For this review, take the finished solid that the model builds, in its own axes (mm). Face numbers are marked on the shaded views. A direction names the side the tool comes from. Give positions to 0.01 mm unless a question says otherwise; leave off trailing zeros. Loops run counter-clockwise (first coordinate to the right, second up) from the corner with the lowest first, then second, coordinate; pieces in that order, holes last. Notation, with made-up numbers: (-33, 2.5) - (23, 2.5) arc R38 cw to (23, 41.5) - close; hole circle Ø7 at (-35.5, 8.25). An arc over 180 degrees is marked (long way). Answer in a Markdown table with one row per item.
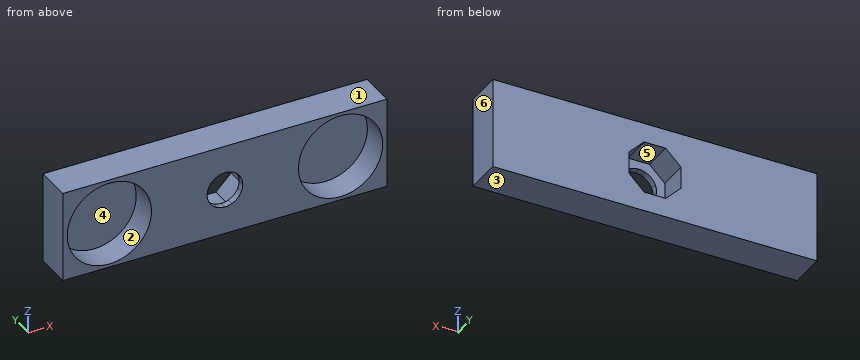
```python
from build123d import *

# Parameters (mm, degrees)
F1_DEPTH = 13.9
F2_DEPTH = 25
F3_R     = 19.5
F4_DEPTH = 17
F6_DEPTH = 20.74372


with BuildPart() as f1:
    # F0 (on Front) → F1 (new body)
    with BuildSketch(Plane.XZ):
        with BuildLine():
            Line((5.0119841047, 12.1), (3.157138317, 7.6220061432))
            ThreePointArc((3.157138317, 7.6220061432), (5.8336309448, 5.8336309448), (7.6220061432, 3.157138317))
            Line((7.6220061432, 3.157138317), (12.1, 5.0119841047))
            Line((12.1, 5.0119841047), (5.0119841047, 12.1))
        make_face()
        with BuildLine():
            Line((0, 12.1), (0, 8.25))
            ThreePointArc((0, 8.25), (1.6094951566, 8.0914785633), (3.157138317, 7.6220061432))
            Line((3.157138317, 7.6220061432), (5.0119841047, 12.1))
            Line((5.0119841047, 12.1), (0, 12.1))
        make_face()
        with BuildLine():
            ThreePointArc((-3.157138317, 7.6220061432), (-1.6094951566, 8.0914785633), (0, 8.25))
            Line((0, 8.25), (0, 12.1))
            Line((0, 12.1), (-5.0119841047, 12.1))
            Line((-5.0119841047, 12.1), (-3.157138317, 7.6220061432))
        make_face()
        with BuildLine():
            ThreePointArc((-7.6220061432, 3.157138317), (-5.8336309448, 5.8336309448), (-3.157138317, 7.6220061432))
            Line((-3.157138317, 7.6220061432), (-5.0119841047, 12.1))
            Line((-5.0119841047, 12.1), (-12.1, 5.0119841047))
            Line((-12.1, 5.0119841047), (-7.6220061432, 3.157138317))
        make_face()
        with BuildLine():
            ThreePointArc((-3.157138317, -7.6220061432), (-5.8336309448, -5.8336309448), (-7.6220061432, -3.157138317))
            Line((-7.6220061432, -3.157138317), (-12.1, -5.0119841047))
            Line((-12.1, -5.0119841047), (-5.0119841047, -12.1))
            Line((-5.0119841047, -12.1), (-3.157138317, -7.6220061432))
        make_face()
        with BuildLine():
            ThreePointArc((-7.6220061432, -3.157138317), (-8.0914785633, -1.6094951566), (-8.25, 0))
            Line((-8.25, 0), (-12.1, 0))
            Line((-12.1, 0), (-12.1, -5.0119841047))
            Line((-12.1, -5.0119841047), (-7.6220061432, -3.157138317))
        make_face()
        with BuildLine():
            Line((-12.1, 0), (-8.25, 0))
            ThreePointArc((-8.25, 0), (-8.0914785633, 1.6094951566), (-7.6220061432, 3.157138317))
            Line((-7.6220061432, 3.157138317), (-12.1, 5.0119841047))
            Line((-12.1, 5.0119841047), (-12.1, 0))
        make_face()
        with BuildLine():
            Line((0, -12.1), (0, -8.25))
            ThreePointArc((0, -8.25), (-1.6094951566, -8.0914785633), (-3.157138317, -7.6220061432))
            Line((-3.157138317, -7.6220061432), (-5.0119841047, -12.1))
            Line((-5.0119841047, -12.1), (0, -12.1))
        make_face()
        with BuildLine():
            ThreePointArc((3.157138317, -7.6220061432), (1.6094951566, -8.0914785633), (0, -8.25))
            Line((0, -8.25), (0, -12.1))
            Line((0, -12.1), (5.0119841047, -12.1))
            Line((5.0119841047, -12.1), (3.157138317, -7.6220061432))
        make_face()
        with BuildLine():
            ThreePointArc((7.6220061432, -3.157138317), (5.8336309448, -5.8336309448), (3.157138317, -7.6220061432))
            Line((3.157138317, -7.6220061432), (5.0119841047, -12.1))
            Line((5.0119841047, -12.1), (12.1, -5.0119841047))
            Line((12.1, -5.0119841047), (7.6220061432, -3.157138317))
        make_face()
        with BuildLine():
            Line((12.1, 0), (8.25, 0))
            ThreePointArc((8.25, 0), (8.0914785633, -1.6094951566), (7.6220061432, -3.157138317))
            Line((7.6220061432, -3.157138317), (12.1, -5.0119841047))
            Line((12.1, -5.0119841047), (12.1, 0))
        make_face()
        with BuildLine():
            ThreePointArc((7.6220061432, 3.157138317), (8.0914785633, 1.6094951566), (8.25, 0))
            Line((8.25, 0), (12.1, 0))
            Line((12.1, 0), (12.1, 5.0119841047))
            Line((12.1, 5.0119841047), (7.6220061432, 3.157138317))
        make_face()
    extrude(amount=F1_DEPTH)


with BuildPart() as f2:
    # F0 (on Front) → F2 (new body)
    with BuildSketch(Plane.XZ):
        with BuildLine():
            Line((3.157138317, 7.6220061432), (0, 0))
            Line((0, 0), (7.6220061432, 3.157138317))
            ThreePointArc((7.6220061432, 3.157138317), (5.8336309448, 5.8336309448), (3.157138317, 7.6220061432))
        make_face()
        with BuildLine():
            Line((0, 8.25), (0, 0))
            Line((0, 0), (3.157138317, 7.6220061432))
            ThreePointArc((3.157138317, 7.6220061432), (1.6094951566, 8.0914785633), (0, 8.25))
        make_face()
        with BuildLine():
            Line((-3.157138317, 7.6220061432), (0, 0))
            Line((0, 0), (0, 8.25))
            ThreePointArc((0, 8.25), (-1.6094951566, 8.0914785633), (-3.157138317, 7.6220061432))
        make_face()
        with BuildLine():
            Line((-7.6220061432, 3.157138317), (0, 0))
            Line((0, 0), (-3.157138317, 7.6220061432))
            ThreePointArc((-3.157138317, 7.6220061432), (-5.8336309448, 5.8336309448), (-7.6220061432, 3.157138317))
        make_face()
        with BuildLine():
            Line((-8.25, 0), (0, 0))
            Line((0, 0), (-7.6220061432, 3.157138317))
            ThreePointArc((-7.6220061432, 3.157138317), (-8.0914785633, 1.6094951566), (-8.25, 0))
        make_face()
        with BuildLine():
            Line((-7.6220061432, -3.157138317), (0, 0))
            Line((0, 0), (-8.25, 0))
            ThreePointArc((-8.25, 0), (-8.0914785633, -1.6094951566), (-7.6220061432, -3.157138317))
        make_face()
        with BuildLine():
            Line((-3.157138317, -7.6220061432), (0, 0))
            Line((0, 0), (-7.6220061432, -3.157138317))
            ThreePointArc((-7.6220061432, -3.157138317), (-5.8336309448, -5.8336309448), (-3.157138317, -7.6220061432))
        make_face()
        with BuildLine():
            Line((0, -8.25), (0, 0))
            Line((0, 0), (-3.157138317, -7.6220061432))
            ThreePointArc((-3.157138317, -7.6220061432), (-1.6094951566, -8.0914785633), (0, -8.25))
        make_face()
        with BuildLine():
            Line((3.157138317, -7.6220061432), (0, 0))
            Line((0, 0), (0, -8.25))
            ThreePointArc((0, -8.25), (1.6094951566, -8.0914785633), (3.157138317, -7.6220061432))
        make_face()
        with BuildLine():
            Line((7.6220061432, -3.157138317), (0, 0))
            Line((0, 0), (3.157138317, -7.6220061432))
            ThreePointArc((3.157138317, -7.6220061432), (5.8336309448, -5.8336309448), (7.6220061432, -3.157138317))
        make_face()
        with BuildLine():
            Line((8.25, 0), (0, 0))
            Line((0, 0), (7.6220061432, -3.157138317))
            ThreePointArc((7.6220061432, -3.157138317), (8.0914785633, -1.6094951566), (8.25, 0))
        make_face()
        with BuildLine():
            Line((7.6220061432, 3.157138317), (0, 0))
            Line((0, 0), (8.25, 0))
            ThreePointArc((8.25, 0), (8.0914785633, 1.6094951566), (7.6220061432, 3.157138317))
        make_face()
    extrude(amount=F2_DEPTH)


with BuildPart() as f4:
    # F3 (on Front) → F4 (new body)
    with BuildSketch(Plane.XZ):
        Polygon((75, 21), (-75, 21), (-75, 0), (-75, -21), (75, -21), (75, 0), align=None)
        with BuildLine():
            ThreePointArc((-34, 0), (-53.5, -19.5), (-73, 0))
            ThreePointArc((-73, 0), (-53.5, 19.5), (-34, 0))
        make_face(mode=Mode.SUBTRACT)
        with Locations((53.5, 0)):
            Circle(F3_R, mode=Mode.SUBTRACT)
        with BuildLine():
            ThreePointArc((-34, 0), (-53.5, 19.5), (-73, 0))
            ThreePointArc((-73, 0), (-53.5, -19.5), (-34, 0))
        make_face()
        with Locations((53.5, 0)):
            Circle(F3_R)
    extrude(amount=F4_DEPTH)

    # F5: cut F2, F1
    add(f2.part, mode=Mode.SUBTRACT)
    add(f1.part, mode=Mode.SUBTRACT)


with BuildPart() as f6:
    # F3 (on Front) → F6 (new body)
    with BuildSketch(Plane.XZ):
        with BuildLine():
            ThreePointArc((-34, 0), (-53.5, 19.5), (-73, 0))
            ThreePointArc((-73, 0), (-53.5, -19.5), (-34, 0))
        make_face()
    extrude(amount=F6_DEPTH)


with BuildPart() as f6b:
    # F3 (on Front) → F6, piece 2 (new body)
    with BuildSketch(Plane.XZ):
        with Locations((53.5, 0)):
            Circle(F3_R)
    extrude(amount=F6_DEPTH)


with BuildPart() as f6_1:
    # F7: moved
    add(f6.part.moved(Location((0, -4, 0))))


with BuildPart() as f6b_1:
    # F7: moved
    add(f6b.part.moved(Location((0, -4, 0))))


with BuildPart() as f4_1:
    add(f4.part)

    # F8: cut F6, F6b
    add(f6_1.part, mode=Mode.SUBTRACT)
    add(f6b_1.part, mode=Mode.SUBTRACT)


solid = f4_1.part
```
1. Wall thickness on line 1 (X direction, y = -6.75, z = 0); line 2 (Z direction, x = -53.5, y = -11.75); line 3 (X direction, y = -14.25, z = -17): over which ranges is each line inside the solid? List them lowest first. Write a range as [from, to].
Values:
| item | result |
|---|---|
| line 1 | x = [-75, -73], [-34, -12.1], [12.1, 34], [73, 75] |
| line 2 | z = [-21, -19.5], [19.5, 21] |
| line 3 | x = [-75, -63.05], [-43.95, 43.95], [63.05, 75] |
2. For the marked faces 4, 5 and 6, list the 3-axis set-ups (+Z, -Z, +X, -X, +Y, -Y) from which the entire face can be reached by the end or side of a thin tool; tool diameter is ignored.
Values:
| item | result |
|---|---|
| face 4 | -Y |
| face 5 | +Y |
| face 6 | +Z, -Z, +X, +Y, -Y |
3. Clearance check with a flat-ended pin moving along its axis: pin 1 (19.5 mm diameter, centred on x = 59, z = 0, fed in from -Y). State where the tip first meets the part, or that it passes through.
Values:
| item | result |
|---|---|
| pin 1 | stops at y = -4 |
4. We need section D-D, the plane x = 41. Give the boundary of the cut face in (y, z), and give its area (3 significant figures).
Values:
| item | result |
|---|---|
| outline | (-17, -21) - (0, -21) - (0, 21) - (-17, 21) - (-17, 14.97) - (-4, 14.97) - (-4, -14.97) - (-17, -14.97) - close |
| area | 325 mm^2 |
5. We need section A-A, the plane y = -10.25. Give the boundary of the cut face in (x, z).
Values:
| item | result |
|---|---|
| outline | (-75, -21) - (75, -21) - (75, 21) - (-75, 21) - close; hole circle Ø39 at (-53.5, 0); hole (-12.1, -5.01) - (-5.01, -12.1) - (5.01, -12.1) - (12.1, -5.01) - (12.1, 5.01) - (5.01, 12.1) - (-5.01, 12.1) - (-12.1, 5.01) - close; hole circle Ø39 at (53.5, 0) |
6. Mouldability with a two-part tool opening along Z and no side actions: class the marked faces 1, 2 and 3 as released by +Z, released by -Z, zero draft, split by the parting line, or undercut.
Values:
| item | result |
|---|---|
| face 1 | released by +Z |
| face 2 | undercut |
| face 3 | released by -Z |
7. We need section C-C, the plane z = 15. Give the boundary of the cut face in (x, y).
Values:
| item | result |
|---|---|
| outline | (-75, -17) - (-65.96, -17) - (-65.96, -4) - (-41.04, -4) - (-41.04, -17) - (41.04, -17) - (41.04, -4) - (65.96, -4) - (65.96, -17) - (75, -17) - (75, 0) - (-75, 0) - close |
8. We need section B-B, the plane x = -53.5. Give the boundary of the cut face in (y, z).
Values:
| item | result |
|---|---|
| outline | (-17, -21) - (0, -21) - (0, 21) - (-17, 21) - (-17, 19.5) - (-4, 19.5) - (-4, -19.5) - (-17, -19.5) - close |
